```python
from build123d import *

# Parameters (mm, degrees)
SKETCH1_R           = 39
SKETCH1_R_2         = 30
BOSS_EXTRUDE1_DEPTH = 10
SKETCH2_R           = 37
SKETCH2_R_2         = 32
CUT_EXTRUDE1_DEPTH  = 1
SKETCH3_R           = 37
SKETCH3_R_2         = 32
CUT_EXTRUDE2_DEPTH  = 1


with BuildPart() as part:
    # Sketch1 → Boss-Extrude1 (new body)
    with BuildSketch(Plane(origin=(0, 0, 0), x_dir=(1, 0, 0), z_dir=(0, 1, 0))):
        Circle(SKETCH1_R)
        Circle(SKETCH1_R_2, mode=Mode.SUBTRACT)
    extrude(amount=BOSS_EXTRUDE1_DEPTH)

    # Sketch2 → Cut-Extrude1 (cut)
    with BuildSketch(Plane(origin=(0, 10, 0), x_dir=(1, 0, 0), z_dir=(0, 1, 0))):
        Circle(SKETCH2_R)
        Circle(SKETCH2_R_2, mode=Mode.SUBTRACT)
    extrude(amount=-CUT_EXTRUDE1_DEPTH, mode=Mode.SUBTRACT)

    # Sketch3 → Cut-Extrude2 (cut)
    with BuildSketch(Plane.XZ):
        Circle(SKETCH3_R)
        Circle(SKETCH3_R_2, mode=Mode.SUBTRACT)
    extrude(amount=-CUT_EXTRUDE2_DEPTH, mode=Mode.SUBTRACT)


solid = part.part
```
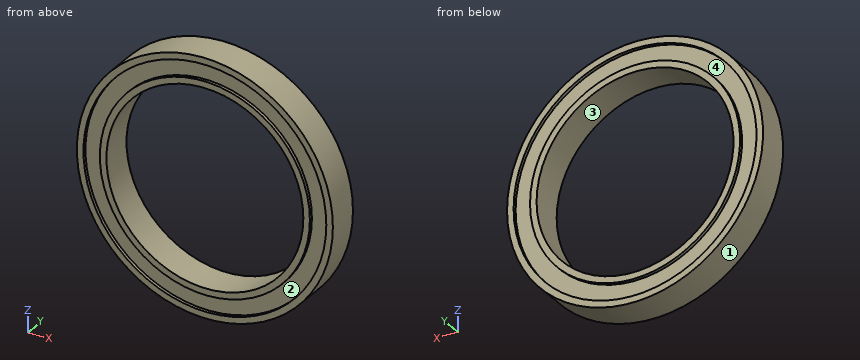
Check sheet for the modelled part. Datum: model origin and axes. Units: mm. Face numbers are marked on the shaded views. A direction names the side the tool comes from. Round coordinates to 2 decimals unless told otherwise and drop trailing zeros. Order: outer loops, then holes, each group sorted by start corner. A loop starts at its lowest first (then second) coordinate and runs counter-clockwise, first axis right, second up.
1) Go/stop test with flat-tipped pins: pin 1 Ø5 at (y, z) = (4, -17) entering from -X; pin 2 Ø4 at (y, z) = (7, 7) entering from -X; pin 3 Ø1 at (y, z) = (6, -22.5) entering from -X. Record where each tip stops, or that it passes through.
2) Mould release check, pull along X, two halves, no side actions. Record for the marked faces 1 and 2: +X half, -X half, draft (parallel to the pull), parting line (faces both ways), or undercut.
3) Section check B-B (x = 0). Record the boundary of the cut face in (y, z).
4) Scan lines: line 1 (X direction, y = 9.45, z = 0); line 2 (Z direction, x = 0, y = 5). Record each from-to range of solid material in increasing order.
5) Section check C-C (y = 2.75). Record the boundary of the cut face in (x, z).
6) Tool access check on the marked faces 3 and 4. Record the directions out of +Z, -Z, +X, -X, +Y, -Y that give a thin tool (end or side, any length) a straight path to the whole face; none if there is none.
7) Section check A-A (z = 0). Record the boundary of the cut face in (x, y).
Result:
1. pin 1: stops at x = -36.2
1. pin 2: stops at x = -38.68
1. pin 3: stops at x = -32.2
2. face 1: parting line
2. face 2: undercut
3. outline: (0, -39) - (10, -39) - (10, -37) - (9, -37) - (9, -32) - (10, -32) - (10, -30) - (0, -30) - (0, -32) - (1, -32) - (1, -37) - (0, -37) - close; (0, 30) - (10, 30) - (10, 32) - (9, 32) - (9, 37) - (10, 37) - (10, 39) - (0, 39) - (0, 37) - (1, 37) - (1, 32) - (0, 32) - close
4. line 1: x = -39 to -37, -32 to -30, 30 to 32, 37 to 39
4. line 2: z = -39 to -30, 30 to 39
5. outline: circle Ø78 at (0, 0); hole circle Ø60 at (0, 0)
6. face 3: +Y, -Y
6. face 4: +Y
7. outline: (-39, 0) - (-37, 0) - (-37, 1) - (-32, 1) - (-32, 0) - (-30, 0) - (-30, 10) - (-32, 10) - (-32, 9) - (-37, 9) - (-37, 10) - (-39, 10) - close; (30, 0) - (32, 0) - (32, 1) - (37, 1) - (37, 0) - (39, 0) - (39, 10) - (37, 10) - (37, 9) - (32, 9) - (32, 10) - (30, 10) - close
